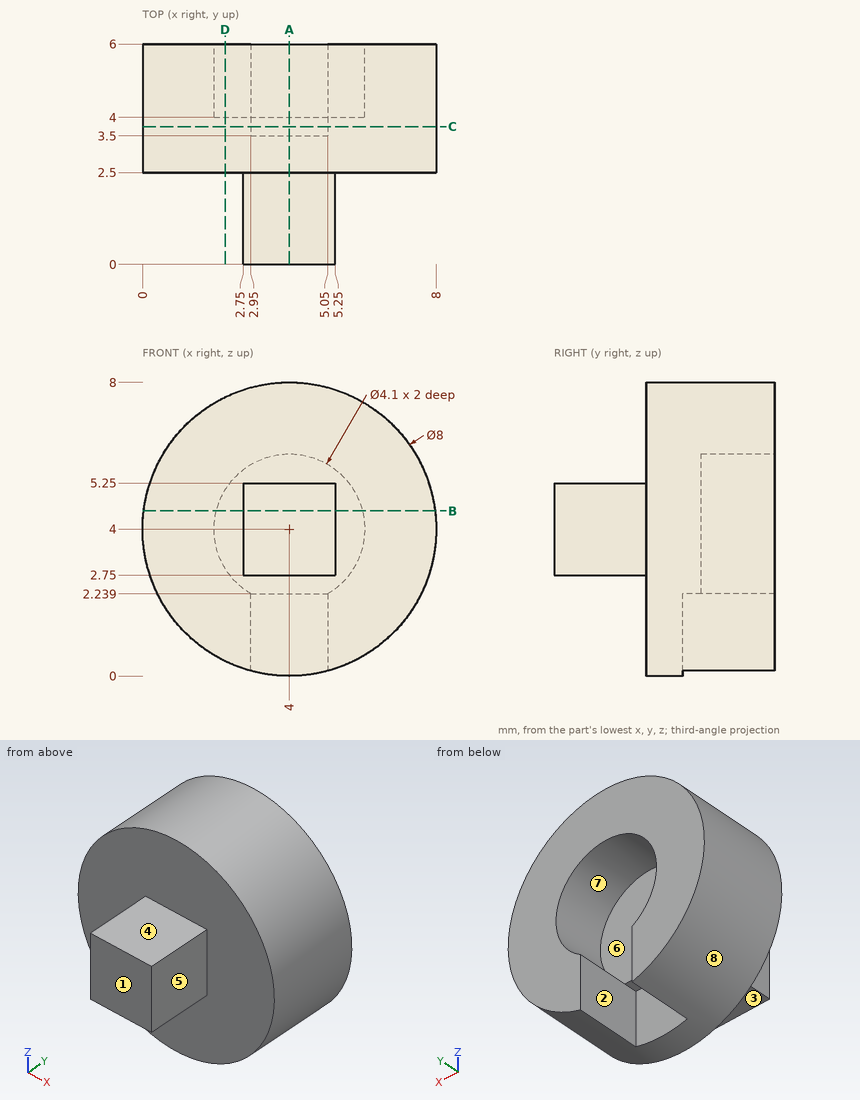
The figure shows three views and two pictorial views of one solid part (mm, origin at its lowest corner). Answer the questions. A direction names the side the tool comes from. Give positions to 0.01 mm unless a question says otherwise; leave off trailing zeros. Order: outer loops, then holes, each group sorted by start corner. A loop starts at its lowest first (then second) coordinate and runs counter-clockwise, first axis right, second up. Notation, with made-up numbers: (-4.5, 45) - (17.5, 45) arc R30 cw to (17.5, 82) - close; hole circle Ø6 at (80.5, -6.75). An arc over 180 degrees is marked (long way). Answer as CSV lines item,"result".
Q1. A cutting plane is placed at C-C, the plane y = 3.75. Determine the outline of the cut face in (x, z).
Answer key:
outline,"(2.95, 0.14) - (2.95, 2.24) - (5.05, 2.24) - (5.05, 0.14) arc R4 ccw (long way) to start"
Q2. Each of these flat-tipped pins is pushed along its axis until it touches: pin 1 Ø0.6 at (x, y) = (4.5, 4) entering from -Z; pin 2 Ø0.8 at (x, y) = (4, 0.5) entering from +Z; pin 3 Ø0.8 at (y, z) = (1, 4.5) entering from +X. Where does it stop, or does it pass through?
Answer key:
pin 1,"stops at z = 2.24"
pin 2,"stops at z = 5.25"
pin 3,"stops at x = 5.25"
Q3. Straight lines are drawn through the part: L1, parallel to X at y = 5.45, z = 4; L2, parallel to Z at x = 4.75, y = 2.2; L3, parallel to Y at x = 4.5, z = 3. For each, find the intervals that lie inside material, in ascending order.
Answer key:
L1,"x = 0 to 1.95, 6.05 to 8"
L2,"z = 2.75 to 5.25"
L3,"y = 0 to 4"
Q4. Which of the six approach directions +Z, -Z, +X, -X, +Y, -Y give full straight-line access (tool end or side, diameter ignored) to the marked faces 1, 2, 3 and 4?
Answer key:
face 1,"+Z, -Z, +X, -X, -Y"
face 2,"-Z, +Y"
face 3,"-Z, +X, -X, -Y"
face 4,"+Z, +X, -X, -Y"
Q5. A cutting plane is placed at D-D, the plane x = 2.25. Determine the outline of the cut face in (y, z).
Answer key:
outline,"(2.5, 0.4) - (6, 0.4) - (6, 2.93) - (4, 2.93) - (4, 5.07) - (6, 5.07) - (6, 7.6) - (2.5, 7.6) - close"
Q6. Determine the mould class of the marked faces 5, 6, 7 and 8 for opening direction X: pulls with the +X half, pulls with the -X half, needs draft (parallel to the pull), parting line crosses it, or undercut.
Answer key:
face 5,"pulls with the +X half"
face 6,"undercut"
face 7,"undercut"
face 8,"parting line crosses it"
Q7. A cutting plane is placed at A-A, the plane x = 4. Determine the outline of the cut face in (y, z).
Answer key:
outline,"(0, 2.75) - (2.5, 2.75) - (2.5, 0) - (3.5, 0) - (3.5, 2.24) - (4, 2.24) - (4, 6.05) - (6, 6.05) - (6, 8) - (2.5, 8) - (2.5, 5.25) - (0, 5.25) - close"
Q8. A cutting plane is placed at B-B, the plane z = 4.5. Determine the outline of the cut face in (x, y).
Answer key:
outline,"(0.03, 2.5) - (2.75, 2.5) - (2.75, 0) - (5.25, 0) - (5.25, 2.5) - (7.97, 2.5) - (7.97, 6) - (5.99, 6) - (5.99, 4) - (2.01, 4) - (2.01, 6) - (0.03, 6) - close"
